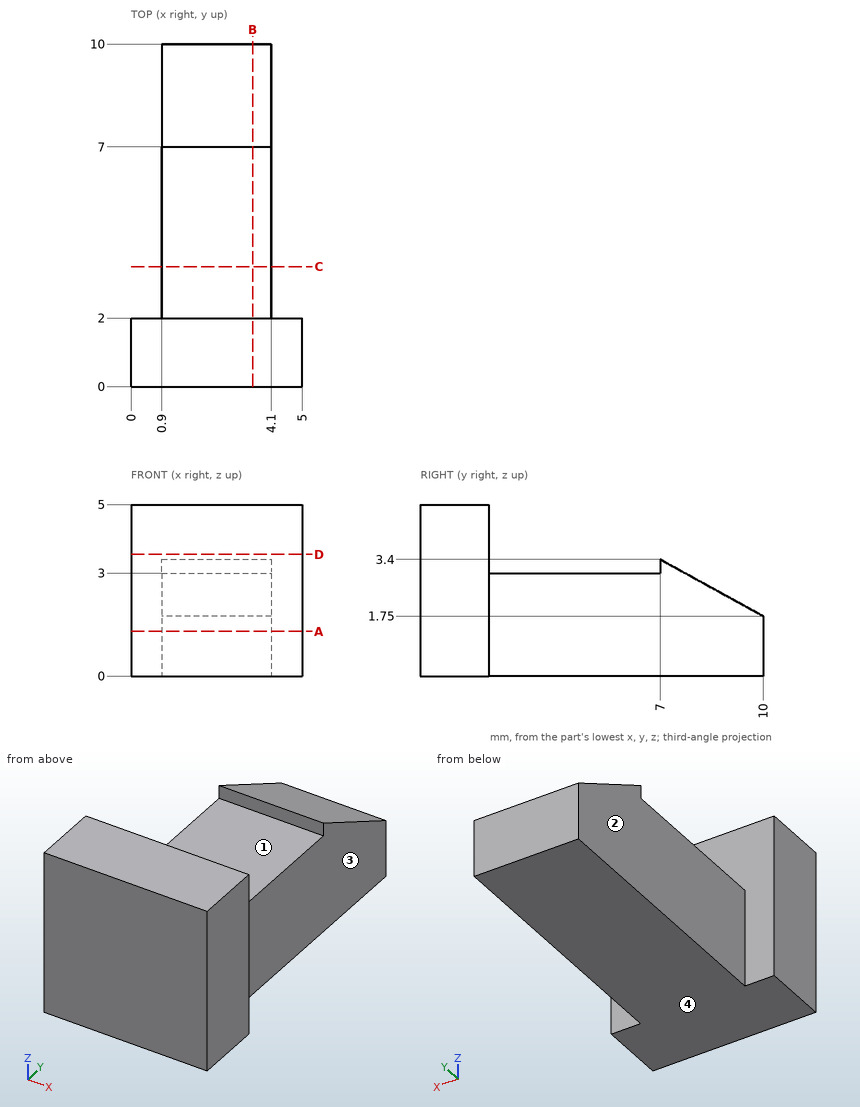
Part print with two shaded views. Sizes in mm from the minimum x, y, z corner. A direction names the side the tool comes from. Round coordinates to 2 decimals unless told otherwise and drop trailing zeros. Order: outer loops, then holes, each group sorted by start corner. A loop starts at its lowest first (then second) coordinate and runs counter-clockwise, first axis right, second up.
(1) 3-axis set-ups, long thin cutter, end or side, ignore diameter. For the marked faces 1, 2, 3 and 4: which of +Z, -Z, +X, -X, +Y, -Y reach the whole face in a straight line?
(2) Band-saw the part on B-B (x = 3.55). List the corners of the cut face in (y, z), then the cut area to 3 significant figures.
(3) Band-saw the part on C-C (y = 3.5). List the corners of the cut face in (x, z), then the cut area to 3 significant figures.
(4) Pin check, flat tips, straight feed: pin 1 (2.5 mm diameter, centred on y = 4.5, z = 1, fed in from -X); pin 2 (2.5 mm diameter, centred on y = 6, z = 2, fed in from +X); pin 3 (2 mm diameter, centred on x = 2.5, y = 4, fed in from +Z). Stop position of each tip, or through.
(5) Band-saw the part on A-A (z = 1.3). List the corners of the cut face in (x, y), then the cut area to 3 significant figures.
(6) Drill centre lines: line 1 (Z direction, x = 1.3, y = 4); line 2 (X direction, y = 4.75, z = 1.55); line 3 (Y direction, x = 0.95, z = 4.2). Where is each one in solid material? Low to high.
(7) Band-saw the part on D-D (z = 3.55). List the corners of the cut face in (x, y).
Verdict:
1. face 1: +Z, +X, -X
1. face 2: +Z, -Z, -X, +Y
1. face 3: +Z, -Z, +X, +Y
1. face 4: -Z, +X, -X, +Y, -Y
2. outline: (0, 0) - (10, 0) - (10, 1.75) - (7, 3.4) - (7, 3) - (2, 3) - (2, 5) - (0, 5) - close
2. area: 32.7 mm2
3. outline: (0.9, 0) - (4.1, 0) - (4.1, 3) - (0.9, 3) - close
3. area: 9.60 mm2
4. pin 1: stops at x = 0.9
4. pin 2: stops at x = 4.1
4. pin 3: stops at z = 3
5. outline: (0, 0) - (5, 0) - (5, 2) - (4.1, 2) - (4.1, 10) - (0.9, 10) - (0.9, 2) - (0, 2) - close
5. area: 35.6 mm2
6. line 1: z = 0 to 3
6. line 2: x = 0.9 to 4.1
6. line 3: y = 0 to 2
7. outline: (0, 0) - (5, 0) - (5, 2) - (0, 2) - close
